Check sheet for the modelled part. Datum: model origin and axes. Units: mm. Face numbers are marked on the shaded views. A direction names the side the tool comes from. Give positions to 0.01 mm unless a question says otherwise; leave off trailing zeros. Order: outer loops, then holes, each group sorted by start corner. A loop starts at its lowest first (then second) coordinate and runs counter-clockwise, first axis right, second up.
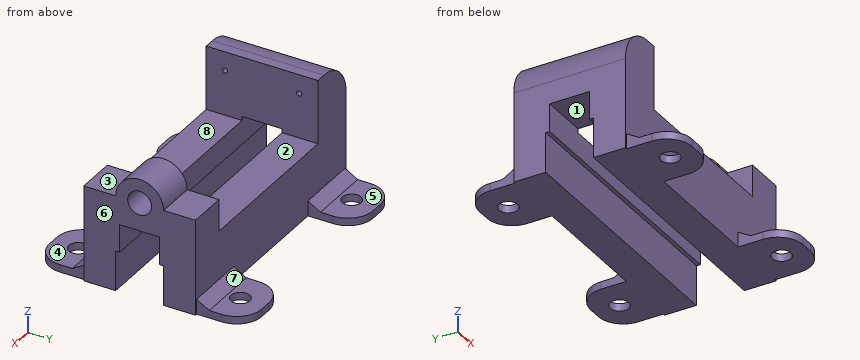
```python
from build123d import *

# Parameters (mm, degrees)
F1_DEPTH  = 88.9
F2_R      = 30
F4_DEPTH  = 31.75
F5_R      = 7.9375
F6_DEPTH  = 55
F7_W      = 15.875
F7_H      = 22.225
F8_DEPTH  = 265
F9_W      = 50
F9_H      = 6
F10_DEPTH = 40
F11_R     = 20
F12_W     = 50
F12_H     = 6
F13_DEPTH = 40
F14_R     = 20
F16_DEPTH = 25
F18_DEPTH = 25
F20_DEPTH = 25
F22_DEPTH = 25
F24_DEPTH = 50
F26_DEPTH = 50
F28_DEPTH = 50
F30_DEPTH = 50
F31_R     = 2
F32_DEPTH = 5
F33_R     = 9.525
F33_R_2   = 7.9375
F34_DEPTH = 78.1


with BuildPart() as f1:
    # F0 (on Front) → F1 (new body)
    with BuildSketch(Plane.XZ):
        Polygon((-86.3789096475, 101.6), (-86.3789096475, 0), (116.8210903525, 0), (116.8210903525, 76.2), (85.0710903525, 76.2), (85.0710903525, 50.8), (-48.2789096475, 50.8), (-48.2789096475, 101.6), align=None)
    extrude(amount=F1_DEPTH)

    # F2
    f2_edges = [f1.edges().sort_by_distance(p)[0] for p in [
        (-86.37891, -44.45, 101.6),
    ]]
    fillet(f2_edges, radius=F2_R)

    # F3 (on face) → F4 (join)
    with BuildSketch(Plane.YZ.offset(116.8210903525)):
        with BuildLine():
            Line((-63.5, 76.2), (-25.4, 76.2))
            ThreePointArc((-25.4, 76.2), (-44.45, 95.25), (-63.5, 76.2))
        make_face()
    extrude(amount=-F4_DEPTH)

    # F5 (on face) → F6 (cut)
    with BuildSketch(Plane.YZ.offset(116.8210903525)):
        with Locations((-44.45, 76.2)):
            Circle(F5_R)
    extrude(amount=-F6_DEPTH, mode=Mode.SUBTRACT)

    # F7 (on face) → F8 (cut)
    with BuildSketch(Plane.YZ.offset(116.8210903525)):
        Polygon((-63.5, 0), (-44.45, 0), (-25.4, 0), (-25.4, 31.75), (-28.575, 31.75), (-44.45, 31.75), (-60.325, 31.75), (-63.5, 31.75), align=None)
        with Locations((-52.3875, 42.8625)):
            Rectangle(F7_W, F7_H)
        with Locations((-36.5125, 42.8625)):
            Rectangle(F7_W, F7_H)
    extrude(amount=-F8_DEPTH, mode=Mode.SUBTRACT)

    # F9 (on face) → F10 (join)
    with BuildSketch(Plane.XZ.offset(88.9)):
        with Locations((-59.7789096475, 3)):
            Rectangle(F9_W, F9_H)
        with Locations((90.2210903525, 3)):
            Rectangle(F9_W, F9_H)
    extrude(amount=F10_DEPTH)

    # F11
    f11_edges = [f1.edges().sort_by_distance(p)[0] for p in [
        (-84.77891, -128.9, 3),
        (-34.77891, -128.9, 3),
        (65.22109, -128.9, 3),
        (115.22109, -128.9, 3),
    ]]
    fillet(f11_edges, radius=F11_R)

    # F12 (on face) → F13 (join)
    with BuildSketch(Plane(origin=(0, 0, 0), x_dir=(-1, 0, 0), z_dir=(0, 1, 0))):
        with Locations((-90.2210903525, 3)):
            Rectangle(F12_W, F12_H)
        with Locations((59.7789096475, 3)):
            Rectangle(F12_W, F12_H)
    extrude(amount=F13_DEPTH)

    # F14
    f14_edges = [f1.edges().sort_by_distance(p)[0] for p in [
        (115.22109, 40, 3),
        (65.22109, 40, 3),
        (-34.77891, 40, 3),
        (-84.77891, 40, 3),
    ]]
    fillet(f14_edges, radius=F14_R)

    # F15 (on face) → F16 (cut)
    with BuildSketch(Plane.XY.offset(6)):
        with BuildLine():
            ThreePointArc((97.7210903525, 20), (95.5243912114, 25.3033008589), (90.2210903525, 27.5))
            ThreePointArc((90.2210903525, 27.5), (84.9177894936, 14.6966991411), (97.7210903525, 20))
        make_face()
    extrude(amount=-F16_DEPTH, mode=Mode.SUBTRACT)

    # F17 (on face) → F18 (cut)
    with BuildSketch(Plane.XY.offset(6)):
        with BuildLine():
            ThreePointArc((-52.2789096475, 20), (-54.4756087886, 25.3033008589), (-59.7789096475, 27.5))
            ThreePointArc((-59.7789096475, 27.5), (-65.0822105064, 14.6966991411), (-52.2789096475, 20))
        make_face()
    extrude(amount=-F18_DEPTH, mode=Mode.SUBTRACT)

    # F19 (on face) → F20 (cut)
    with BuildSketch(Plane.XY.offset(6)):
        with BuildLine():
            ThreePointArc((-52.2789096475, -108.9), (-65.0822105064, -103.5966991411), (-59.7789096475, -116.4))
            ThreePointArc((-59.7789096475, -116.4), (-54.4756087886, -114.2033008589), (-52.2789096475, -108.9))
        make_face()
    extrude(amount=-F20_DEPTH, mode=Mode.SUBTRACT)

    # F21 (on face) → F22 (cut)
    with BuildSketch(Plane.XY.offset(6)):
        with BuildLine():
            ThreePointArc((97.7210903525, -108.9), (84.9177894936, -103.5966991411), (90.2210903525, -116.4))
            ThreePointArc((90.2210903525, -116.4), (95.5243912114, -114.2033008589), (97.7210903525, -108.9))
        make_face()
    extrude(amount=-F22_DEPTH, mode=Mode.SUBTRACT)

    # F23 (on face) → F24 (join)
    with BuildSketch(Plane(origin=(-84.7789096475, 0, 0), x_dir=(0, -1, 0), z_dir=(-1, 0, 0))):
        Polygon((88.9, 6), (98.9, 6), (88.9, 12), align=None)
    extrude(amount=-F24_DEPTH)

    # F25 (on face) → F26 (join)
    with BuildSketch(Plane.YZ.offset(115.2210903525)):
        Polygon((-88.9, 12), (-98.9, 6), (-88.9, 6), align=None)
    extrude(amount=-F26_DEPTH)

    # F27 (on face) → F28 (join)
    with BuildSketch(Plane.YZ.offset(115.2210903525)):
        Polygon((0, 6), (10, 6), (0, 12), align=None)
    extrude(amount=-F28_DEPTH)

    # F29 (on face) → F30 (join)
    with BuildSketch(Plane(origin=(-84.7789096475, 0, 0), x_dir=(0, -1, 0), z_dir=(-1, 0, 0))):
        Polygon((0, 12), (-10, 6), (0, 6), align=None)
    extrude(amount=-F30_DEPTH)

    # F31 (on face) → F32 (cut)
    with BuildSketch(Plane.YZ.offset(-48.2789096475)):
        with BuildLine():
            ThreePointArc((-71.9, 86.6), (-73.9, 88.6), (-75.9, 86.6))
            ThreePointArc((-75.9, 86.6), (-73.9, 84.6), (-71.9, 86.6))
        make_face()
        with Locations((-15, 86.6)):
            Circle(F31_R)
    extrude(amount=-F32_DEPTH, mode=Mode.SUBTRACT)

    # F33 (on face) → F34 (cut)
    with BuildSketch(Plane.YZ.offset(116.8210903525)):
        with Locations((-44.45, 76.2)):
            Circle(F33_R)
        with Locations((-44.45, 76.2)):
            Circle(F33_R_2, mode=Mode.SUBTRACT)
    extrude(amount=-F34_DEPTH, mode=Mode.SUBTRACT)


solid = f1.part
```
(1) Set-up check for the marked faces 1, 2, 3, 4 and 5: record each of +Z, -Z, +X, -X, +Y, -Y from which the full face is reachable in a straight line by a thin tool's end or side.
Response values:
face 1: -Z, +X, -X
face 2: +Z, +Y, -Y
face 3: +Z, +X, -Y
face 4: +Z, +X, -X, -Y
face 5: +Z, +X, -X, +Y
(2) Release check for a two-part mould opening along X. For the marked faces 6, 7 and 8 record: released by +X, released by -X, zero draft, split by the parting line, or undercut.
Response values:
face 6: released by +X
face 7: zero draft
face 8: undercut
(3) Cross-section at D-D on y = -91.5. Enter the section's corners in (x, z).
Response values:
outline: (-84.78, 0) - (-34.78, 0) - (-34.78, 10.44) - (-84.78, 10.44) - close; (65.22, 0) - (115.22, 0) - (115.22, 10.44) - (65.22, 10.44) - close
(4) Cross-section at A-A on y = -44.45. Enter the section's corners in (x, z) (3 decimals).
Response values:
outline: (-86.379, 53.975) - (-48.279, 53.975) - (-48.279, 101.6) - (-56.379, 101.6) arc R30 ccw to (-86.379, 71.6) - close; (85.071, 53.975) - (116.821, 53.975) - (116.821, 66.675) - (85.071, 66.675) - close; (85.071, 85.725) - (116.821, 85.725) - (116.821, 95.25) - (85.071, 95.25) - close
(5) Cross-section at C-C on x = -10. Enter the section's corners in (y, z) (3 decimals), then the cut area to 3 significant figures.
Response values:
outline: (-88.9, 0) - (-63.5, 0) - (-63.5, 31.75) - (-60.325, 31.75) - (-60.325, 50.8) - (-88.9, 50.8) - close; (-28.575, 31.75) - (-25.4, 31.75) - (-25.4, 0) - (0, 0) - (0, 50.8) - (-28.575, 50.8) - close
area: 2,700 mm2
(6) Material ranges on L1, parallel to X at y = -108, z = 2; L2, parallel to Y at x = -55, z = 53.5 (3 decimals); L3, parallel to Z at x = 103, y = -44 (3 decimals), recorded low to high.
Response values:
L1: x = -84.78 to -67.22, -52.33 to -34.78, 65.22 to 82.78, 97.67 to 115.22
L2: y = -88.9 to -60.325, -28.575 to 0
L3: z = 53.975 to 66.686, 85.714 to 95.245
(7) Gauge pin test, flat ends, axial feed: pin 1 Ø8 at (x, z) = (95, 90.5) entering from -Y; pin 2 Ø8.5 at (x, y) = (39, -21.5) entering from +Z; pin 3 Ø13 at (y, z) = (-101, 4) entering from +X. Record the tip position at first contact, or that the pin passes through.
Response values:
pin 1: stops at y = -60.48
pin 2: stops at z = 50.8
pin 3: stops at x = 115.22
(8) Cross-section at B-B on z = 19. Enter the section's corners in (x, y), then the cut area to 3 significant figures.
Response values:
outline: (-86.38, -88.9) - (116.82, -88.9) - (116.82, -63.5) - (-86.38, -63.5) - close; (-86.38, -25.4) - (116.82, -25.4) - (116.82, 0) - (-86.38, 0) - close
area: 10,300 mm2
